```python
from build123d import *

# Parameters (mm, degrees)
F0_W     = 755.65
F0_H     = 292.1
F1_DEPTH = 800.1
F2_W     = 692.456603
F2_H     = 359.491945
F3_DEPTH = 266.7
F4_W     = 692.456603
F4_H     = 322.354048
F5_DEPTH = 266.7


with BuildPart() as f1:
    # F0 (on Top) → F1 (new body)
    with BuildSketch(Plane.XY):
        with Locations((2.138129, -21.109734)):
            Rectangle(F0_W, F0_H)
    extrude(amount=F1_DEPTH)

    # F2 (on face) → F3 (cut)
    with BuildSketch(Plane.XZ.offset(167.159734)):
        with Locations((2.476693, 207.432329)):
            Rectangle(F2_W, F2_H)
    extrude(amount=-F3_DEPTH, mode=Mode.SUBTRACT)

    # F4 (on face) → F5 (cut)
    with BuildSketch(Plane.XZ.offset(167.159734)):
        with Locations((2.476693, 580.808595)):
            Rectangle(F4_W, F4_H)
    extrude(amount=-F5_DEPTH, mode=Mode.SUBTRACT)


solid = f1.part
```
Input: part model. Units: mm. Frame: model coordinates. A direction names the side the tool comes from. Coordinates: 2 decimals unless noted, no trailing zeros. Loops run counter-clockwise (first coordinate to the right, second up) from the corner with the lowest first, then second, coordinate; pieces in that order, holes last. Notation, with made-up numbers: M -27,61.25 L -1,61.25 A33 ccw -1,93.25 Z; hole C 34.5,-20.75 d9. An arc over 180 degrees is marked long. Use a Markdown table: item, result. Add a question column.
1) Section C-C, the plane z = 223. Return the cut outline in (x, y) (3 decimals), plus the area to 3 significant figures.
2) Section B-B, the plane x = 31.5. Return the cut outline in (y, z).
3) Set-up query: faces 1 (the flat face through (0, -167.16, 398)), 2 (the flat face through (-2, -36, 387.178)). Return all of +Z, -Z, +X, -X, +Y, -Y with unobstructed straight access to the full face (end or side cutting, diameter ignored); none if empty.
4) Line query: L1, parallel to Z at x = 129.5, y = -100.5; L2, parallel to X at y = -84.5, z = 646 (3 decimals); L3, parallel to Y at x = -131.5, z = 499.5. Output: solid intervals per line, ascending. Write a range as from..to.
5) Draft query along Z for faces 3 (the flat face through (-3, -19, 800.1)), 4 (the flat face through (-343.752, -36, 205)), 5 (the flat face through (379.963, -23, 394)), 6 (the flat face through (-3, -19, 0)). Return one class per face: +Z half, -Z half, draft (parallel to the pull), parting line (faces both ways), or undercut.
6) Pin query (flat end, axial travel): P1, Ø10, axis at x = 203.5, z = 639, coming from the -Y side. Return the tip coordinate at first contact, or that it passes through.
7) Section A-A, the plane y = -121.5. Return the cut outline in (x, z) (3 decimals).
Answer below:
| question | item | result |
|---|---|---|
| 1 | outline | M -375.687,-167.16 L -343.752,-167.16 L -343.752,99.54 L 348.705,99.54 L 348.705,-167.16 L 379.963,-167.16 L 379.963,124.94 L -375.687,124.94 Z |
| 1 | area | 36,000 mm2 |
| 2 | outline | M -167.16,0 L 124.94,0 L 124.94,800.1 L -167.16,800.1 L -167.16,741.99 L 99.54,741.99 L 99.54,419.63 L -167.16,419.63 L -167.16,387.18 L 99.54,387.18 L 99.54,27.69 L -167.16,27.69 Z |
| 3 | face 1 | +Z, -Z, +X, -X, -Y |
| 3 | face 2 | -Y |
| 4 | L1 | 0..27.69, 387.18..419.63, 741.99..800.1 |
| 4 | L2 | -375.687..-343.752, 348.705..379.963 |
| 4 | L3 | 99.54..124.94 |
| 5 | face 3 | +Z half |
| 5 | face 4 | undercut |
| 5 | face 5 | draft |
| 5 | face 6 | -Z half |
| 6 | P1 | y = 99.54 |
| 7 | outline | M -375.687,0 L 379.963,0 L 379.963,800.1 L -375.687,800.1 Z; hole M -343.752,27.686 L 348.705,27.686 L 348.705,387.178 L -343.752,387.178 Z; hole M -343.752,419.632 L 348.705,419.632 L 348.705,741.986 L -343.752,741.986 Z |
